Source: CAD feature listing. Evaluate the final solid. Frame: model axes, mm. Give positions to 0.01 mm unless a question says otherwise; leave off trailing zeros. Loops run counter-clockwise (first coordinate to the right, second up) from the corner with the lowest first, then second, coordinate; pieces in that order, holes last. Notation, with made-up numbers: M 62.5,-18 L 107.5,-18 A29 ccw 107.5,21 Z; hole C 66.5,0.25 d11. An arc over 180 degrees is marked long. Put each result on its own line as item: value. Start each with the question number.
Autodesk Inventor part; units mm, degrees
ref_plane "YZ Plane" through (0, 0, 0) normal (1, 0, 0) x (0, 1, 0)
ref_plane "XZ Plane" through (0, 0, 0) normal (0, 1, 0) x (-1, 0, 0)
ref_plane "XY Plane" through (0, 0, 0) normal (0, 0, 1) x (1, 0, 0)
sketch "Sketch1" plane through (0, 0, 0) normal (0, 0, 1) x (1, 0, 0)
  circle A0 centre (0, 0) radius 142.621
  circle A1 centre (0, 0) radius 132.461
  point P0 (0, 137.541)
  point P1 (-119.114, 68.7705)
  point P2 (-119.114, -68.7705)
  point P3 (0, -137.541)
  point P4 (119.114, -68.7705)
  point P5 (119.114, 68.7705)
  dimension "d0" = 285.242
  dimension "d1" = 264.922
  dimension "d2" = 137.541
  dimension "d5" = 360
extrude "Extrusion1" add sketch "Sketch1" against normal blind 6.096
hole "Hole1" at (0, 137.541, 0) at (-119.114, 68.7705, 0) at (-119.114, -68.7705, 0) at (0, -137.541, 0) at (119.114, -68.7705, 0) at (119.114, 68.7705, 0) direction (0, 0, -1) diameter 6.35 depth 25.4 tip angle 118
properties part number "inner piece"
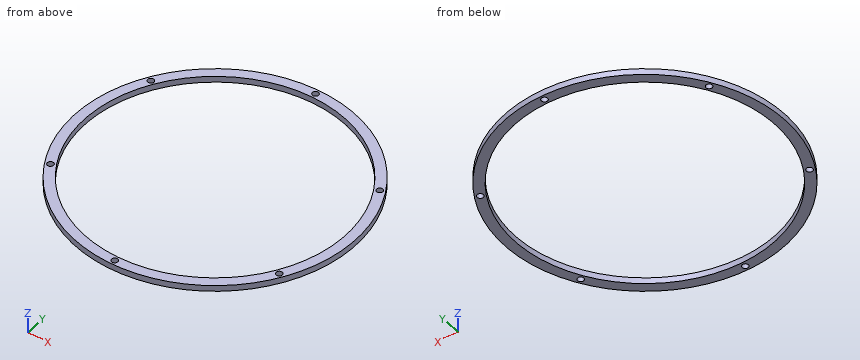
1. Section C-C, the plane z = -3.5. State how many separate pieces and enclosed holes the cut face has, plus the area to 3 significant figures.
2. Section A-A, the plane y = 0. Output: boundary loops of the cut face in (x, z), plus the area to 3 significant figures.
3. Contact query for flat-ended pins moving along their axis: pin 1 (5.5 mm diameter, centred on x = -119.11, y = 68.77, fed in from +Z); pin 2 (1 mm diameter, centred on y = 34.5, z = -3, fed in from +X); pin 3 (1 mm diameter, centred on x = -4.5, z = -5, fed in from -Y); pin 4 (3 mm diameter, centred on x = 102.5, z = -5, fed in from +Y). Output: stop coordinate, or through.
4. Section B-B, the plane x = -80.5. Output: boundary loops of the cut face in (y, z), plus the area to 3 significant figures.
5. Ray query, line 1 (Y direction, x = 0, z = -2.5); line 2 (Y direction, x = -69, z = -5); line 3 (X direction, y = 120, z = -0.5). Return the intervals inside material, ascending.
Results found:
1. separate pieces: 1
1. enclosed holes: 7
1. area: 8,590 mm²
2. outline: M -142.62,-6.1 L -132.46,-6.1 L -132.46,0 L -142.62,0 Z; M 132.46,-6.1 L 142.62,-6.1 L 142.62,0 L 132.46,0 Z
2. area: 124 mm²
3. pin 1: through
3. pin 2: x = 138.51
3. pin 3: y = -142.56
3. pin 4: y = 100.7
4. outline: M -117.73,-6.1 L -105.19,-6.1 L -105.19,0 L -117.73,0 Z; M 105.19,-6.1 L 117.73,-6.1 L 117.73,0 L 105.19,0 Z
4. area: 153 mm²
5. line 1: -142.62 to -140.72, -134.37 to -132.46, 132.46 to 134.37, 140.72 to 142.62
5. line 2: -124.82 to -113.07, 113.07 to 124.82
5. line 3: -77.08 to -56.09, 56.09 to 77.08
